Part model, mm, in its own coordinate system. Face numbers are marked on the shaded views. Give positions to 0.01 mm unless a question says otherwise; leave off trailing zeros. Write each loop counter-clockwise with the first axis right and the second up, starting at its lowest first coordinate (ties: lowest second). Pieces come first, ordered by that corner, then holes.
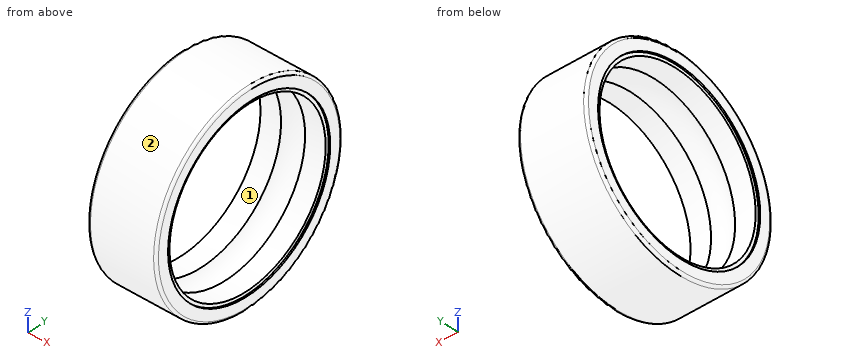
Autodesk Inventor part; units mm, degrees
ref_plane "mss_or_XY" through (0, 0, 0) normal (1, 0, 0) x (0, 0, -1)
ref_plane "mss_or_YZ" through (0, 0, 0) normal (0, 0, -1) x (0, 1, 0)
ref_plane "mss_or_ZX" through (0, 0, 0) normal (0, 1, 0) x (1, 0, 0)
sketch "Sketch_3" plane through (0, 0, 0) normal (0, 0, 1) x (1, 0, 0)
  line L0 (4, 0) -> (0, 0)
  line L1 (0, 5.232) -> (0.09, 5.232)
  line L2 (0.09, 5.232) -> (0.09, 5.04)
  line L3 (0.09, 5.04) -> (1.2951, 5.04)
  arc A0 (2.7049, 5.04) -> (1.2951, 5.04) centre (2, 4.5) ccw
  line L4 (2.7049, 5.04) -> (3.91, 5.04)
  line L5 (3.91, 5.04) -> (3.91, 5.232)
  line L6 (3.91, 5.232) -> (4, 5.232)
  line L7 (4, 5.232) -> (4, 5.85)
  arc A1 (4, 5.85) -> (3.85, 6) centre (3.85, 5.85) ccw
  line L8 (3.85, 6) -> (0.15, 6)
  arc A2 (0.15, 6) -> (0, 5.85) centre (0.15, 5.85) ccw
  line L9 (0, 5.85) -> (0, 5.232)
revolve "Revolution1" add sketch "Sketch_3" angle 360 about axis through (4, 0, 0) along (1, 0, 0)
ref_plane "mss_or_XY" through (0, 0, 0) normal (1, 0, 0) x (0, 0, -1)
ref_plane "mss_or_YZ" through (0, 0, 0) normal (0, 0, -1) x (0, 1, 0)
ref_plane "mss_or_ZX" through (0, 0, 0) normal (0, 1, 0) x (1, 0, 0)
ref_plane "mss_or11_XY" through (4, 0, 0) normal (1, 0, 0) x (0, 0, -1)
ref_plane "mss_or11_YZ" through (4, 0, 0) normal (0, 0, -1) x (0, 1, 0)
ref_plane "mss_or11_ZX" through (4, 0, 0) normal (0, 1, 0) x (1, 0, 0)
ref_plane "mss_or2_1_XY" through (1.5, 4.5, 0) normal (1, 0, 0) x (0, 0, -1)
ref_plane "mss_or2_1_YZ" through (1.5, 4.5, 0) normal (0, 0, -1) x (0, 1, 0)
ref_plane "mss_or2_1_ZX" through (1.5, 4.5, 0) normal (0, 1, 0) x (1, 0, 0)
ref_plane "mss_or2_2_XY" through (1.5, 3.4472, 2.8925) normal (1, 0, 0) x (0, 0, -1)
ref_plane "mss_or2_2_YZ" through (1.5, 3.4472, 2.8925) normal (0, 0, -1) x (0, 1, 0)
ref_plane "mss_or2_2_ZX" through (1.5, 3.4472, 2.8925) normal (0, 1, 0) x (1, 0, 0)
ref_plane "mss_or2_3_XY" through (1.5, 0.7814, 4.4316) normal (1, 0, 0) x (0, 0, -1)
ref_plane "mss_or2_3_YZ" through (1.5, 0.7814, 4.4316) normal (0, 0, -1) x (0, 1, 0)
ref_plane "mss_or2_3_ZX" through (1.5, 0.7814, 4.4316) normal (0, 1, 0) x (1, 0, 0)
ref_plane "mss_or2_4_XY" through (1.5, -2.25, 3.8971) normal (1, 0, 0) x (0, 0, -1)
ref_plane "mss_or2_4_YZ" through (1.5, -2.25, 3.8971) normal (0, 0, -1) x (0, 1, 0)
ref_plane "mss_or2_4_ZX" through (1.5, -2.25, 3.8971) normal (0, 1, 0) x (1, 0, 0)
ref_plane "mss_or2_5_XY" through (1.5, -4.2286, 1.5391) normal (1, 0, 0) x (0, 0, -1)
ref_plane "mss_or2_5_YZ" through (1.5, -4.2286, 1.5391) normal (0, 0, -1) x (0, 1, 0)
ref_plane "mss_or2_5_ZX" through (1.5, -4.2286, 1.5391) normal (0, 1, 0) x (1, 0, 0)
ref_plane "mss_or2_6_XY" through (1.5, -4.2286, -1.5391) normal (1, 0, 0) x (0, 0, -1)
ref_plane "mss_or2_6_YZ" through (1.5, -4.2286, -1.5391) normal (0, 0, -1) x (0, 1, 0)
ref_plane "mss_or2_6_ZX" through (1.5, -4.2286, -1.5391) normal (0, 1, 0) x (1, 0, 0)
ref_plane "mss_or2_7_XY" through (1.5, -2.25, -3.8971) normal (1, 0, 0) x (0, 0, -1)
ref_plane "mss_or2_7_YZ" through (1.5, -2.25, -3.8971) normal (0, 0, -1) x (0, 1, 0)
ref_plane "mss_or2_7_ZX" through (1.5, -2.25, -3.8971) normal (0, 1, 0) x (1, 0, 0)
ref_plane "mss_or2_8_XY" through (1.5, 0.7814, -4.4316) normal (1, 0, 0) x (0, 0, -1)
ref_plane "mss_or2_8_YZ" through (1.5, 0.7814, -4.4316) normal (0, 0, -1) x (0, 1, 0)
ref_plane "mss_or2_8_ZX" through (1.5, 0.7814, -4.4316) normal (0, 1, 0) x (1, 0, 0)
ref_plane "mss_or2_9_XY" through (1.5, 3.4472, -2.8925) normal (1, 0, 0) x (0, 0, -1)
ref_plane "mss_or2_9_YZ" through (1.5, 3.4472, -2.8925) normal (0, 0, -1) x (0, 1, 0)
ref_plane "mss_or2_9_ZX" through (1.5, 3.4472, -2.8925) normal (0, 1, 0) x (1, 0, 0)
ref_plane "mss_or21_1_XY" through (2, 4.5, 0) normal (1, 0, 0) x (0, 0, -1)
ref_plane "mss_or21_1_YZ" through (2, 4.5, 0) normal (0, 0, -1) x (0, 1, 0)
ref_plane "mss_or21_1_ZX" through (2, 4.5, 0) normal (0, 1, 0) x (1, 0, 0)
ref_plane "mss_or21_2_XY" through (2, 3.4472, 2.8925) normal (1, 0, 0) x (0, 0, -1)
ref_plane "mss_or21_2_YZ" through (2, 3.4472, 2.8925) normal (0, 0, -1) x (0, 1, 0)
ref_plane "mss_or21_2_ZX" through (2, 3.4472, 2.8925) normal (0, 1, 0) x (1, 0, 0)
ref_plane "mss_or21_3_XY" through (2, 0.7814, 4.4316) normal (1, 0, 0) x (0, 0, -1)
ref_plane "mss_or21_3_YZ" through (2, 0.7814, 4.4316) normal (0, 0, -1) x (0, 1, 0)
ref_plane "mss_or21_3_ZX" through (2, 0.7814, 4.4316) normal (0, 1, 0) x (1, 0, 0)
ref_plane "mss_or21_4_XY" through (2, -2.25, 3.8971) normal (1, 0, 0) x (0, 0, -1)
ref_plane "mss_or21_4_YZ" through (2, -2.25, 3.8971) normal (0, 0, -1) x (0, 1, 0)
ref_plane "mss_or21_4_ZX" through (2, -2.25, 3.8971) normal (0, 1, 0) x (1, 0, 0)
ref_plane "mss_or21_5_XY" through (2, -4.2286, 1.5391) normal (1, 0, 0) x (0, 0, -1)
ref_plane "mss_or21_5_YZ" through (2, -4.2286, 1.5391) normal (0, 0, -1) x (0, 1, 0)
ref_plane "mss_or21_5_ZX" through (2, -4.2286, 1.5391) normal (0, 1, 0) x (1, 0, 0)
ref_plane "mss_or21_6_XY" through (2, -4.2286, -1.5391) normal (1, 0, 0) x (0, 0, -1)
ref_plane "mss_or21_6_YZ" through (2, -4.2286, -1.5391) normal (0, 0, -1) x (0, 1, 0)
ref_plane "mss_or21_6_ZX" through (2, -4.2286, -1.5391) normal (0, 1, 0) x (1, 0, 0)
ref_plane "mss_or21_7_XY" through (2, -2.25, -3.8971) normal (1, 0, 0) x (0, 0, -1)
ref_plane "mss_or21_7_YZ" through (2, -2.25, -3.8971) normal (0, 0, -1) x (0, 1, 0)
ref_plane "mss_or21_7_ZX" through (2, -2.25, -3.8971) normal (0, 1, 0) x (1, 0, 0)
ref_plane "mss_or21_8_XY" through (2, 0.7814, -4.4316) normal (1, 0, 0) x (0, 0, -1)
ref_plane "mss_or21_8_YZ" through (2, 0.7814, -4.4316) normal (0, 0, -1) x (0, 1, 0)
ref_plane "mss_or21_8_ZX" through (2, 0.7814, -4.4316) normal (0, 1, 0) x (1, 0, 0)
ref_plane "mss_or21_9_XY" through (2, 3.4472, -2.8925) normal (1, 0, 0) x (0, 0, -1)
ref_plane "mss_or21_9_YZ" through (2, 3.4472, -2.8925) normal (0, 0, -1) x (0, 1, 0)
ref_plane "mss_or21_9_ZX" through (2, 3.4472, -2.8925) normal (0, 1, 0) x (1, 0, 0)
properties part number "WBC6-12ZZ Outer ring"
1) Saw through at C-C, the plane x = 0.4. Write the cut outline in (y, z), then the cut area to 3 significant figures.
Answers follow:
outline: circle Ø12 at (0, 0); hole circle Ø10.08 at (0, 0)
area: 33.3 mm2
2) Saw through at A-A, the plane y = 0. Write the cut outline in (x, z), then the cut area to 3 significant figures.
Answers follow:
outline: (0, -5.85) arc R0.15 ccw to (0.15, -6) - (3.85, -6) arc R0.15 ccw to (4, -5.85) - (4, -5.23) - (3.91, -5.23) - (3.91, -5.04) - (2.7, -5.04) arc R0.89 cw to (1.3, -5.04) - (0.09, -5.04) - (0.09, -5.23) - (0, -5.23) - close; (0, 5.23) - (0.09, 5.23) - (0.09, 5.04) - (1.3, 5.04) arc R0.89 cw to (2.7, 5.04) - (3.91, 5.04) - (3.91, 5.23) - (4, 5.23) - (4, 5.85) arc R0.15 ccw to (3.85, 6) - (0.15, 6) arc R0.15 ccw to (0, 5.85) - close
area: 6.91 mm2
3) Pin check, flat tip, straight feed: pin 1 Ø2 at (y, z) = (-3.5, -1.5) entering from -X. Stop position of the tip, or through.
Answers follow:
pin 1: passes through
4) Wall check: L1, parallel to Z at x = 3.6, y = 0; L2, parallel to Z at x = 2.4, y = 3.25; L3, parallel to Y at x = 3.25, z = 2. Give the ranges that are in metal, low to high.
Answers follow:
L1: z = -6 to -5.04, 5.04 to 6
L2: z = -5.04 to -4.18, 4.18 to 5.04
L3: y = -5.66 to -4.63, 4.63 to 5.66
5) Two-plate mould, pull along Y, no slides. Class the marked faces 1 and 2: +Y half, -Y half, draft (parallel to the pull), parting line (faces both ways), or undercut.
Answers follow:
face 1: undercut
face 2: parting line
6) Saw through at D-D, the plane x = 2.5. Write the cut outline in (y, z), then the cut area to 3 significant figures.
Answers follow:
outline: circle Ø12 at (0, 0); hole circle Ø10.47 at (0, 0)
area: 27.0 mm2
